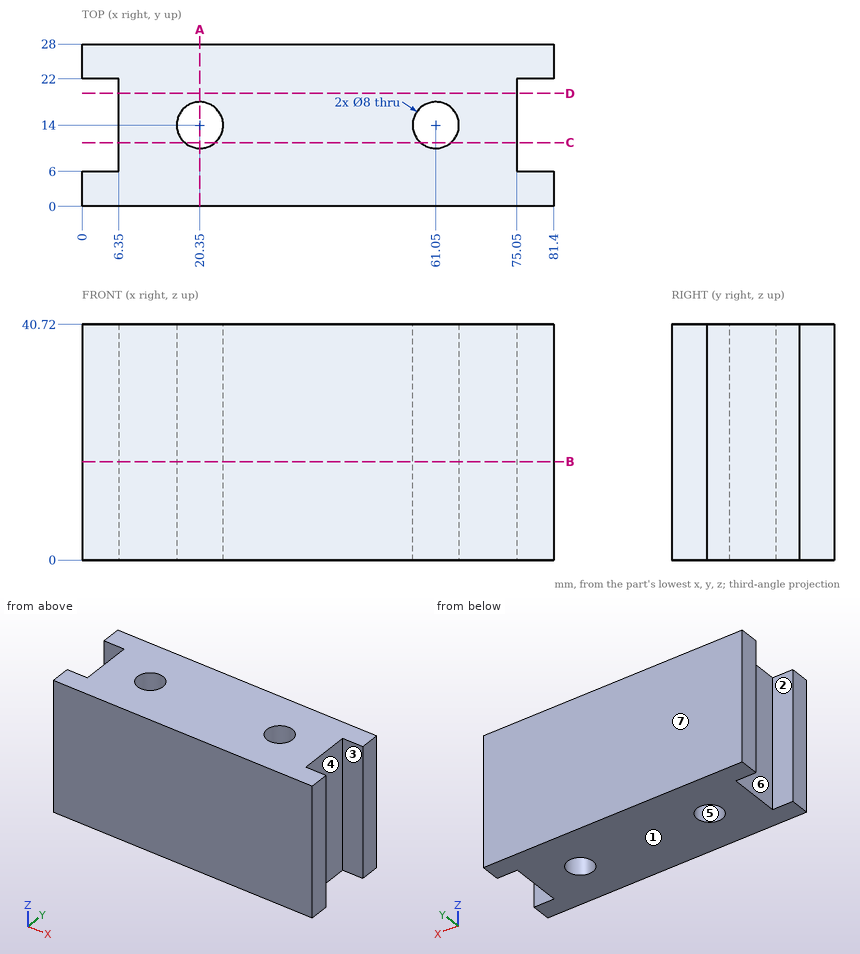
Source: three-view drawing plus pictorial views. Frame: mm from the lowest corner of the part. A direction names the side the tool comes from. Coordinates: 2 decimals unless noted, no trailing zeros. Loops run counter-clockwise (first coordinate to the right, second up) from the corner with the lowest first, then second, coordinate; pieces in that order, holes last. Notation, with made-up numbers: (-10.75, 60.25) - (20.25, 60.25) arc R28 cw to (20.25, 84.25) - close; hole circle Ø11 at (67.25, -22.75). An arc over 180 degrees is marked (long way). One line per question, with ' | ' between items.
1) Set-up query: the marked faces 1, 2 and 3. Return all of +Z, -Z, +X, -X, +Y, -Y with unobstructed straight access to the full face (end or side cutting, diameter ignored); none if empty.
Report:
face 1: -Z, +X, -X, +Y, -Y | face 2: +Z, -Z, -X | face 3: +Z, -Z, +X
2) Section B-B, the plane z = 17. Return loops of the section in (x, y).
Report:
outline: (0, 0) - (81.4, 0) - (81.4, 6) - (75.05, 6) - (75.05, 22) - (81.4, 22) - (81.4, 28) - (0, 28) - (0, 22) - (6.35, 22) - (6.35, 6) - (0, 6) - close; hole circle Ø8 at (20.35, 14); hole circle Ø8 at (61.05, 14)
3) Section C-C, the plane y = 11. Return loops of the section in (x, z), then the cut area to 3 significant figures.
Report:
outline: (6.35, 0) - (17.7, 0) - (17.7, 40.72) - (6.35, 40.72) - close; (23, 0) - (58.4, 0) - (58.4, 40.72) - (23, 40.72) - close; (63.7, 0) - (75.05, 0) - (75.05, 40.72) - (63.7, 40.72) - close | area: 2,370 mm²
4) First-contact query: P1, Ø7, axis at x = 20.35, y = 14, coming from the -Z side; P2, Ø13, axis at y = 13.5, z = 14, coming from the -X side; P3, Ø3, axis at y = 14.5, z = 35, coming from the +X side. Flat tips, straight axial feed; report the tip coordinate or a pass-through.
Report:
P1: passes through | P2: stops at x = 6.35 | P3: stops at x = 75.05
5) Section D-D, the plane y = 19.5. Return loops of the section in (x, z).
Report:
outline: (6.35, 0) - (75.05, 0) - (75.05, 40.72) - (6.35, 40.72) - close
6) Line query: line 1 along X through (y, z) = (14.25, 32.5); line 2 along Y through (x, z) = (61.05, 32.5); line 3 along X through (y, z) = (13, 27.5). Output: solid intervals per line, ascending.
Report:
line 1: x = 6.35 to 16.36, 24.34 to 57.06, 65.04 to 75.05 | line 2: y = 0 to 10, 18 to 28 | line 3: x = 6.35 to 16.48, 24.22 to 57.18, 64.92 to 75.05
7) Pull-direction query (X, two-part tool) for the marked faces 4, 5, 6 and 7; classes: released by +X, released by -X, zero draft, split by the parting line, or undercut.
Report:
face 4: released by +X | face 5: undercut | face 6: released by -X | face 7: zero draft
8) Section A-A, the plane x = 20.35. Return loops of the section in (y, z), then the cut area to 3 significant figures.
Report:
outline: (0, 0) - (10, 0) - (10, 40.72) - (0, 40.72) - close; (18, 0) - (28, 0) - (28, 40.72) - (18, 40.72) - close | area: 814 mm²
